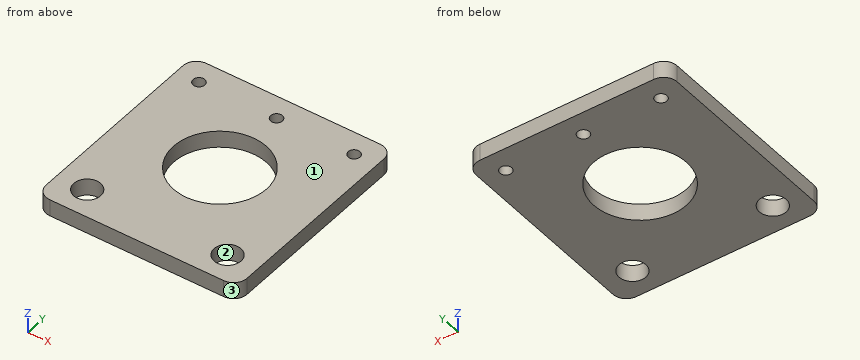
from build123d import *

# Parameters (mm, degrees)
SKETCH1_W           = 37.9349
SKETCH1_H           = 37.9349
BOSS_EXTRUDE1_DEPTH = 3.175
SKETCH9_R           = 1.1176
SKETCH9_R_2         = 2.54
SKETCH9_R_3         = 8.763
CUT_EXTRUDE2_DEPTH  = 3.175
SKETCH11_W          = 37.9349
SKETCH11_H          = 3.175
BOSS_EXTRUDE2_DEPTH = 2.54
FILLET1_R           = 2.54


with BuildPart() as part:
    # Sketch1 → Boss-Extrude1 (new body)
    with BuildSketch(Plane.XY):
        with Locations((18.96745, 18.96745)):
            Rectangle(SKETCH1_W, SKETCH1_H)
    extrude(amount=BOSS_EXTRUDE1_DEPTH)

    # Sketch9 → Cut-Extrude2 (cut)
    with BuildSketch(Plane.XY.offset(3.175)):
        with Locations((33.62325, 33.62325)):
            Circle(SKETCH9_R)
        with Locations((4.31165, 33.62325)):
            Circle(SKETCH9_R)
        with Locations((5.70865, 2.78765)):
            Circle(SKETCH9_R_2)
        with Locations((32.22625, 2.78765)):
            Circle(SKETCH9_R_2)
        with Locations((18.96745, 33.62325)):
            Circle(SKETCH9_R)
        with Locations((18.96745, 18.96745)):
            Circle(SKETCH9_R_3)
    extrude(amount=-CUT_EXTRUDE2_DEPTH, mode=Mode.SUBTRACT)

    # Sketch11 → Boss-Extrude2 (add)
    with BuildSketch(Plane.XZ):
        with Locations((18.96745, 1.5875)):
            Rectangle(SKETCH11_W, SKETCH11_H)
    extrude(amount=BOSS_EXTRUDE2_DEPTH)

    # Fillet1
    fillet1_edges = [part.edges().sort_by_distance(p)[0] for p in [
        (0, -2.54, 1.5875),
        (37.9349, -2.54, 1.5875),
        (0, 37.9349, 1.5875),
        (37.9349, 37.9349, 1.5875),
    ]]
    fillet(fillet1_edges, radius=FILLET1_R)


solid = part.part
For this review, take the finished solid that the model builds, in its own axes (mm). Face numbers are marked on the shaded views. Give positions to 0.01 mm unless a question says otherwise; leave off trailing zeros. Loops run counter-clockwise (first coordinate to the right, second up) from the corner with the lowest first, then second, coordinate; pieces in that order, holes last. Notation, with made-up numbers: M 86,86.5 L 98,86.5 A5 cw 98,92.5 Z; hole C 40,-36 d11. An arc over 180 degrees is marked long. Put each result on its own line as item: value. Start each with the question number.
(1) Add section D-D, the plane z = 1.55. Write out the cut boundary in (x, y).
(2) Add section A-A, the plane y = 12.5. Write out the cut boundary in (x, z) (3 decimals), then the cut area to 3 significant figures.
(3) Add section B-B, the plane x = 25.5. Write out the cut boundary in (y, z) (3 decimals), then the cut area to 3 significant figures.
(4) The part is to be moulded in two halves that separate along X. For the marked faces 1, 2 and 3, say which applies: +X half, -X half, draft (parallel to the pull), parting line (faces both ways), or undercut.
(5) Wall thickness on L1, parallel to X at y = 19, z = 0.2; L2, parallel to Y at x = 33.5, z = 1.55; L3, parallel to X at y = 0.5, z = 1.55: over which ranges is each line inside the solid? List them lowest first.
(6) Add section C-C, the plane y = 4. Write out the cut boundary in (x, z) (3 decimals), then the cut area to 3 significant figures.
Result:
1. outline: M 0,0 A2.54 ccw 2.54,-2.54 L 35.39,-2.54 A2.54 ccw 37.93,0 L 37.93,35.39 A2.54 ccw 35.39,37.93 L 2.54,37.93 A2.54 ccw 0,35.39 Z; hole C 5.71,2.79 d5.08; hole C 4.31,33.62 d2.24; hole C 18.97,18.97 d17.53; hole C 18.97,33.62 d2.24; hole C 32.23,2.79 d5.08; hole C 33.62,33.62 d2.24
2. outline: M 0,0 L 13.055,0 L 13.055,3.175 L 0,3.175 Z; M 24.88,0 L 37.935,0 L 37.935,3.175 L 24.88,3.175 Z
2. area: 82.9 mm^2
3. outline: M -2.54,0 L 13.127,0 L 13.127,3.175 L -2.54,3.175 Z; M 24.808,0 L 37.935,0 L 37.935,3.175 L 24.808,3.175 Z
3. area: 91.4 mm^2
4. face 1: draft
4. face 2: undercut
4. face 3: +X half
5. L1: x = 0 to 10.2, 27.73 to 37.93
5. L2: y = -2.54 to 0.59, 4.99 to 32.51, 34.73 to 37.93
5. L3: x = 0 to 4.6, 6.81 to 31.12, 33.33 to 37.93
6. outline: M 0,0 L 3.477,0 L 3.477,3.175 L 0,3.175 Z; M 7.941,0 L 29.994,0 L 29.994,3.175 L 7.941,3.175 Z; M 34.458,0 L 37.935,0 L 37.935,3.175 L 34.458,3.175 Z
6. area: 92.1 mm^2
